Autodesk Inventor part; units mm, degrees
ref_plane "Work Plane8" through (0, 5, 0) normal (0, 1, 0) x (1, 0, 0)
ref_plane "YZ Plane" through (0, 0, 0) normal (1, 0, 0) x (0, 1, 0)
ref_plane "XZ Plane" through (0, 0, 0) normal (0, 1, 0) x (-1, 0, 0)
sketch "Sketch1" plane through (0, 0, 0) normal (0, 1, 0) x (-1, 0, 0)
  line L0 (30, 30) -> (-30, 30)
  line L1 (-30, 30) -> (-30, -30)
  line L2 (-30, -30) -> (30, -30)
  line L3 (30, -30) -> (30, 30)
  line L4 (30, 30) -> (-30, -30) construction
  line L5 (-30, 30) -> (30, -30) construction
  point P0 (0, 0)
  dimension "d0" = 60
  dimension "d1" = 60
extrude "Extrusion1" add sketch "Sketch1" along normal blind 10
fillet "Fillet1" radius 7 4 edges at (30, 5, 30) (30, 5, -30) (-30, 5, 30) (-30, 5, -30)
sketch "Sketch2" plane through (0, 10, 0) normal (0, 1, 0) x (1, 0, 0)
  line L0 (-30, 30) -> (30, 30)
  line L1 (30, 30) -> (30, -30)
  line L2 (30, -30) -> (-30, -30)
  line L3 (-30, -30) -> (-30, 30)
  line L4 (-30, 30) -> (30, -30) construction
  line L5 (30, 30) -> (-30, -30) construction
  line L6 (25, -25) -> (25, 25)
  line L7 (25, 25) -> (-25, 25)
  line L8 (-25, 25) -> (-25, -25)
  line L9 (-25, -25) -> (25, -25)
  circle A0 centre (25, -25) radius 2.75
  circle A1 centre (-25, -25) radius 2.75
  circle A2 centre (25, 25) radius 2.75
  circle A3 centre (-25, 25) radius 2.75
  point P0 (0, 0)
  dimension "d5" = 5
  dimension "d6" = 5.5
  dimension "d7" = 5.5
  dimension "d8" = 5.5
  dimension "d9" = 5.5
extrude "Extrusion2" cut sketch "Sketch2" against normal blind 3 contours L9 A0 L6 | L6 A0 L9 | A2 L7 L6 | L6 L7 A2 | A1 L8 L9 | L9 L8 A1 | A3 L8 L7 | L7 L8 A3
sketch "Sketch7" plane through (0, 10, 0) normal (0, 1, 0) x (1, 0, 0)
  line L0 (-23, 30) -> (23, 30)
  line L1 (30, 23) -> (30, -23)
  line L2 (23, -30) -> (-23, -30)
  line L3 (-30, -23) -> (-30, 23)
  line L4 (-30, 30) -> (30, -30) construction
  line L5 (30, 30) -> (-30, -30) construction
  arc A0 (-23, 30) -> (-30, 23) centre (-23, 23) ccw
  arc A1 (-30, -23) -> (-23, -30) centre (-23, -23) ccw
  arc A2 (23, -30) -> (30, -23) centre (23, -23) ccw
  arc A3 (30, 23) -> (23, 30) centre (23, 23) ccw
  line L6 (23, 32) -> (-23, 32)
  arc A4 (-23, 32) -> (-32, 23) centre (-23, 23) ccw
  line L7 (-32, 23) -> (-32, -23)
  arc A5 (-32, -23) -> (-23, -32) centre (-23, -23) ccw
  line L8 (-23, -32) -> (23, -32)
  arc A6 (23, -32) -> (32, -23) centre (23, -23) ccw
  line L9 (32, -23) -> (32, 23)
  arc A7 (32, 23) -> (23, 32) centre (23, 23) ccw
  point P0 (0, 0)
  dimension "d47" = 7
  dimension "d48" = 2
extrude "Extrusion6" add sketch "Sketch7" against normal blind 10
sketch "Sketch30" plane through (0, 10, 0) normal (0, 1, 0) x (1, 0, 0)
  line L0 (-25, -25) -> (25, -25)
  line L1 (25, -25) -> (25, 25)
  line L2 (25, 25) -> (-25, 25)
  line L3 (-25, 25) -> (-25, -25)
  line L4 (-25, -25) -> (25, 25) construction
  line L5 (25, -25) -> (-25, 25) construction
  line L6 (21, 21) -> (21, -21)
  line L7 (21, -21) -> (-21, -21)
  line L8 (-21, -21) -> (-21, 21)
  line L9 (-21, 21) -> (21, 21)
  line L10 (-13.4, 21) -> (-13.4, -2.8)
  line L11 (-13.4, -2.8) -> (21, -2.8)
  line L12 (19, -19) -> (-19, -19)
  line L13 (-19, -19) -> (-19, 19)
  line L14 (-11.4, 19) -> (-11.4, -0.8)
  line L15 (-11.4, -0.8) -> (19, -0.8)
  line L16 (-11.4, 19) -> (19, 19)
  line L17 (19, 19) -> (19, -0.8)
  point P0 (0, 0)
  dimension "d307" = 50
  dimension "d308" = 50
  dimension "d309" = 4
  dimension "d310" = 34.4
  dimension "d311" = 23.8
  dimension "d313" = 2
extrude "Extrusion28" cut sketch "Sketch30" against normal blind 2 contours L6 L11 L10 L9
sketch "Sketch31" plane through (0, 10, 0) normal (0, 1, 0) x (1, 0, 0)
  line L0 (-11.4, 19) -> (19, 19)
  line L1 (19, 19) -> (19, -0.8)
  line L2 (19, -0.8) -> (-11.4, -0.8)
  line L3 (-11.4, -0.8) -> (-11.4, 19)
  point P0 (0, 0)
extrude "Extrusion29" cut sketch "Sketch31" against normal blind 8
sketch "Sketch32" plane through (0, 10, 0) normal (0, 1, 0) x (1, 0, 0)
  line L0 (32, -23) -> (32, 23)
  line L1 (23, 32) -> (-23, 32)
  line L2 (-13.4, 21) -> (21, 21)
  line L3 (-32, 23) -> (-32, -23)
  line L4 (-18, 28) -> (18, 28)
  line L5 (18, 28) -> (18, 25)
  line L6 (18, 25) -> (-18, 25)
  line L7 (-18, 25) -> (-18, 28)
  line L8 (-23, -32) -> (23, -32)
  line L9 (21, 21) -> (21, -2.8)
  line L10 (28, 18) -> (25, 18)
  line L11 (25, 18) -> (25, -18)
  line L12 (25, -18) -> (28, -18)
  line L13 (28, -18) -> (28, 18)
  line L14 (21, -2.8) -> (-13.4, -2.8)
  line L15 (18, -28) -> (-18, -28)
  line L16 (-18, -28) -> (-18, -6.8)
  line L17 (-18, -6.8) -> (21, -6.8)
  line L18 (21, -6.8) -> (21, -18)
  line L19 (21, -18) -> (18, -18)
  line L20 (18, -18) -> (18, -28)
  line L21 (-13.4, -2.8) -> (-13.4, 21)
  line L22 (-22, -18) -> (-28, -18)
  line L23 (-28, -18) -> (-28, 18)
  line L24 (-28, 18) -> (-17.4, 18)
  line L25 (-17.4, 18) -> (-17.4, -2.8)
  line L26 (-17.4, -2.8) -> (-22, -2.8)
  line L27 (-22, -2.8) -> (-22, -18)
  point P0 (0, 0)
  dimension "d318" = 14
  dimension "d319" = 4
  dimension "d320" = 4
  dimension "d321" = 4
  dimension "d322" = 14
  dimension "d323" = 4
  dimension "d324" = 14
  dimension "d325" = 4
  dimension "d326" = 14
  dimension "d327" = 4
  dimension "d328" = 14
  dimension "d329" = 4
  dimension "d330" = 4
  dimension "d331" = 4
  dimension "d332" = 14
  dimension "d333" = 4
  dimension "d334" = 14
  dimension "d335" = 4
  dimension "d336" = 14
  dimension "d337" = 4
  dimension "d338" = 4
  dimension "d339" = 4
  dimension "d341" = 4
  dimension "d342" = 14
  dimension "d343" = 14
extrude "Extrusion30" cut sketch "Sketch32" against normal through all contours L4 L5 L6 L7 | L13 L12 L11 L10 | L15 L16 L17 L18 L19 L20 | L22 L23 L24 L25 L26 L27
fillet "Fillet9" radius 0.5 8 edges at (-18, 5, -28) (25, 5, -18) (25, 5, 18) (-18, 5, -25) (18, 5, -25) (28, 5, 18) (18, 5, -28) (28, 5, -18)
fillet "Fillet9" radius 1 10 edges at (3.8, 2, -19) (3.8, 2, 0.8) (19, 2, -9.1) (-11.4, 2, -9.1) (18, 5, 18) (21, 5, 18) (-22, 5, 2.8) (-17.4, 5, 2.8) (-22, 5, 18) (-28, 5, 18)
fillet "Fillet9" radius 2 6 edges at (-28, 5, -18) (-17.4, 5, -18) (21, 5, 6.8) (-18, 5, 28) (-18, 5, 6.8) (18, 5, 28)
ref_plane "Work Plane8" through (0, 5, 0) normal (0, 1, 0) x (1, 0, 0)
mirror "Mirror8" about plane through (0, 5, 0) normal (0, 1, 0) of "Extrusion2"
properties part number "8 pin long"
Check sheet for the modelled part. Datum: model origin and axes. Units: mm. A direction names the side the tool comes from. Round coordinates to 2 decimals unless told otherwise and drop trailing zeros. Order: outer loops, then holes, each group sorted by start corner. A loop starts at its lowest first (then second) coordinate and runs counter-clockwise, first axis right, second up.
1) Section check D-D (z = 25). Record the boundary of the cut face in (x, y), and give its area (3 significant figures).
2) Section check B-B (x = -2). Record the boundary of the cut face in (y, z).
3) Scan lines: line 1 (X direction, y = 3.25, z = 10); line 2 (X direction, y = 7.5, z = -11); line 3 (Z direction, x = 12, y = 5.5). Record each from-to range of solid material in increasing order.
4) Mould release check, pull along X, two halves, no side actions. Record for faces 4 (the flat face through (-32, 5, 0)), 5 (the flat face through (0, 5, 32)), 6 (the flat face through (0, 5, -25)): +X half, -X half, draft (parallel to the pull), parting line (faces both ways), or undercut.
5) Section check C-C (y = 4). Give the number of separate pieces and of enclosed holes in the cut face, and give its area (3 significant figures).
6) Go/stop test with flat-tipped pins: pin 1 Ø3 at (x, z) = (25.5, 25) entering from +Y; pin 2 Ø3 at (x, z) = (-24, 25) entering from -Y. Record where each tip stops, or that it passes through.
7) Section check A-A (z = 5). Record the boundary of the cut face in (x, y), and give its area (3 significant figures).
8) Tool access check on faces 1 (the flat face through (-15, 10, -8)), 2 (the flat face through (-25, 7, 25)), 3 (the flat face through (1, 5, 6.8)). Record the directions out of +Z, -Z, +X, -X, +Y, -Y that give a thin tool (end or side, any length) a straight path to the whole face; none if there is none.
Result:
1. outline: (-31.77, 0) - (-27.75, 0) - (-27.75, 3) - (-22.25, 3) - (-22.25, 0) - (-18, 0) - (-18, 10) - (-22.25, 10) - (-22.25, 7) - (-27.75, 7) - (-27.75, 10) - (-31.77, 10) - close; (18, 0) - (22.25, 0) - (22.25, 3) - (27.75, 3) - (27.75, 0) - (31.77, 0) - (31.77, 10) - (27.75, 10) - (27.75, 7) - (22.25, 7) - (22.25, 10) - (18, 10) - close
1. area: 209 mm2
2. outline: (0, -32) - (10, -32) - (10, -28) - (0, -28) - close; (0, -25) - (10, -25) - (10, -21) - (8, -21) - (8, -19) - (3, -19) arc R1 cw to (2, -18) - (2, -0.2) arc R1 cw to (3, 0.8) - (8, 0.8) - (8, 2.8) - (10, 2.8) - (10, 6.8) - (0, 6.8) - close; (0, 28) - (10, 28) - (10, 32) - (0, 32) - close
3. line 1: x = -32 to -28, -22 to -18, 21 to 25, 28 to 32
3. line 2: x = -32 to -28, -17.4 to -11.4, 19 to 25, 28 to 32
3. line 3: z = -32 to -28, -25 to -19, 0.8 to 6.8, 28 to 32
4. face 4: -X half
4. face 5: draft
4. face 6: undercut
5. separate pieces: 1
5. enclosed holes: 5
5. area: 2,110 mm2
6. pin 1: stops at y = 7
6. pin 2: stops at y = 3
7. outline: (-32, 0) - (-28, 0) - (-28, 10) - (-32, 10) - close; (-22, 0) - (25, 0) - (25, 10) - (-22, 10) - close; (28, 0) - (32, 0) - (32, 10) - (28, 10) - close
7. area: 550 mm2
8. face 1: +Z, -Z, +X, -X, +Y
8. face 2: +Y
8. face 3: +Y, -Y
